```python
from build123d import *

# Parameters (mm, degrees)
SKETCH_W        = 82
SKETCH_H        = 70
PAD_DEPTH       = 2
SKETCH001_W     = 2
SKETCH001_H     = 7
PAD001_DEPTH    = 2
SKETCH011_W     = 8
SKETCH011_H     = 6.8
PAD002_DEPTH    = 4
SKETCH012_W     = 7
SKETCH012_H     = 6
PAD003_DEPTH    = 4
SKETCH010_W     = 8
SKETCH010_H     = 6.8
PAD004_DEPTH    = 4
SKETCH013_R     = 1.15
POCKET_DEPTH    = 80.001
SKETCH016_R     = 1.15
POCKET001_DEPTH = 8.501
SKETCH018_W     = 11.5
SKETCH018_H     = 11.5
POCKET002_DEPTH = 5
POCKET003_DEPTH = 5
POCKET004_DEPTH = 5
SKETCH021_W     = 1
SKETCH021_H     = 7
PAD005_DEPTH    = 1
SKETCH022_W     = 9
SKETCH022_H     = 10
POCKET005_DEPTH = 0.4
FILLET_R        = 2


with BuildPart() as part:
    # Sketch → Pad (new body)
    with BuildSketch(Plane.XY):
        Rectangle(SKETCH_W, SKETCH_H)
    extrude(amount=PAD_DEPTH)

    # Sketch001 (on Face6 of Pad) → Pad001 (join)
    with BuildSketch(Plane.XY.offset(2)):
        with Locations((-38, 0)):
            Rectangle(SKETCH001_W, SKETCH001_H)
        Polygon((-21, 33), (39, 33), (39, -4), (37, -4), (37, 31), (-21, 31), align=None)
    extrude(amount=PAD001_DEPTH)

    # Sketch011 (on Face15 of Pad001) → Pad002 (join)
    with BuildSketch(Plane.YZ.offset(39)):
        with Locations((0, 5.4)):
            Rectangle(SKETCH011_W, SKETCH011_H)
    extrude(amount=-PAD002_DEPTH)

    # Sketch012 (on Face9 of Pad002) → Pad003 (join)
    with BuildSketch(Plane(origin=(-39, 0, 0), x_dir=(0, -1, 0), z_dir=(-1, 0, 0))):
        with Locations((0, 5)):
            Rectangle(SKETCH012_W, SKETCH012_H)
    extrude(amount=-PAD003_DEPTH)

    # Sketch010 (on Face16 of Pad001) → Pad004 (join)
    with BuildSketch(Plane(origin=(0, 33, 0), x_dir=(-1, 0, 0), z_dir=(0, 1, 0))):
        with Locations((-29, 5.4)):
            Rectangle(SKETCH010_W, SKETCH010_H)
        with Locations((14, 5.4)):
            Rectangle(SKETCH010_W, SKETCH010_H)
    extrude(amount=-PAD004_DEPTH)

    # Sketch013 (on Face44 of Pad004) → Pocket (cut, through all)
    with BuildSketch(Plane.YZ.offset(39)):
        with Locations((0, 5)):
            Circle(SKETCH013_R)
    extrude(amount=-POCKET_DEPTH, mode=Mode.SUBTRACT)

    # Sketch016 → Pocket001 (cut, through all)
    with BuildSketch(Plane.XZ.offset(-26.5)):
        with Locations((-14, 5)):
            Circle(SKETCH016_R)
        with Locations((29, 5)):
            Circle(SKETCH016_R)
    extrude(amount=-POCKET001_DEPTH, mode=Mode.SUBTRACT)

    # Sketch018 (on Face5 of Pocket001) → Pocket002 (cut)
    with BuildSketch(Plane.XY.offset(2)):
        with Locations((0, 17.75)):
            Rectangle(SKETCH018_W, SKETCH018_H)
    extrude(amount=-POCKET002_DEPTH, mode=Mode.SUBTRACT)

    # Sketch019 (on Face31 of Pocket002) → Pocket003 (cut)
    with BuildSketch(Plane.XZ.offset(-29)):
        Polygon((29.125944, 9.042901), (33.258869, 4.499726), (33.258869, 9.042901), align=None)
    extrude(amount=-POCKET003_DEPTH, mode=Mode.SUBTRACT)

    # Sketch020 (on Face36 of Pocket003) → Pocket004 (cut)
    with BuildSketch(Plane(origin=(35, 0, 0), x_dir=(0, -1, 0), z_dir=(-1, 0, 0))):
        Polygon((2.77547, 8.938441), (6.386171, 3.079567), (6.386171, 8.938441), align=None)
    extrude(amount=-POCKET004_DEPTH, mode=Mode.SUBTRACT)

    # Sketch021 (on Face40 of Pocket004) → Pad005 (join)
    with BuildSketch(Plane.XY.offset(8)):
        with Locations((-38.5, 0)):
            Rectangle(SKETCH021_W, SKETCH021_H)
    extrude(amount=PAD005_DEPTH)

    # Sketch022 (on Face5 of Pocket003) → Pocket005 (cut)
    with BuildSketch(Plane.XY.offset(2)):
        with Locations((-29.3, 30)):
            Rectangle(SKETCH022_W, SKETCH022_H)
    extrude(amount=-POCKET005_DEPTH, mode=Mode.SUBTRACT)

    # Fillet
    fillet_edges = [part.edges().sort_by_distance(p)[0] for p in [
        (41, 35, 1),
        (-41, 35, 1),
    ]]
    fillet(fillet_edges, radius=FILLET_R)


solid = part.part
```
The model under review builds one solid part; all positions refer to its coordinate system, in mm. A direction names the side the tool comes from. Round coordinates to 2 decimals unless told otherwise and drop trailing zeros. Loops run counter-clockwise (first coordinate to the right, second up) from the corner with the lowest first, then second, coordinate; pieces in that order, holes last.
1) Consider section A-A on x = -14. State the section outline as (y, z) points, then the cut area to 3 significant figures.
Values follow:
outline: (-35, 0) - (35, 0) - (35, 2) - (33, 2) - (33, 3.85) - (29, 3.85) - (29, 2) - (-35, 2) - close; (29, 6.15) - (33, 6.15) - (33, 8.8) - (29, 8.8) - close
area: 158 mm2
2) The part is to be moulded in two halves that separate along Y. For faces 1 (the face through (37, 4, 6)), 2 (the face through (40.4, 34.43, 1.01)), 3 (the face through (8, 32, 4)), say which applies: pulls with the +Y half, pulls with the -Y half, needs draft (parallel to the pull), parting line crosses it, or undercut.
Values follow:
face 1: undercut
face 2: pulls with the +Y half
face 3: needs draft
3) Tool access review of faces 4 (the face through (35, 1, 6)), 5 (the face through (5.75, 18, 1)), 6 (the face through (-19, 32, 4)), 7 (the face through (-29, 30, 1.6)): name each direction out of +Z, -Z, +X, -X, +Y, -Y from which nothing blocks a thin tool from reaching the whole face with its end or side.
Values follow:
face 4: +Z, -Y
face 5: +Z, -Z
face 6: +Z, -X, +Y, -Y
face 7: +Z, +Y
4) Clearance check with flat-ended pins moving along their axes: P1, Ø5, axis at x = -0.5, z = 7.5, coming from the -Y side; P2, Ø1, axis at y = 13.5, z = 3, coming from the -X side; P3, Ø3.5, axis at y = 0, z = 5, coming from the +X side; P4, Ø4.5, axis at x = -16, y = 30.5, coming from the +Z side. State where each tip first meets the part, or that it passes through.
Values follow:
P1: passes through
P2: stops at x = 37
P3: stops at x = 39
P4: stops at z = 8.8
5) Consider section C-C on x = 24. State the section outline as (y, z) points.
Values follow:
outline: (-35, 0) - (35, 0) - (35, 2) - (33, 2) - (33, 4) - (31, 4) - (31, 2) - (-35, 2) - close
6) Wall thickness on line 1 along Z through (x, y) = (-37.75, 0); line 2 along Z through (x, y) = (37.8, 0); line 3 along Y through (x, z) = (-12.5, 4): over which ranges is each line inside the solid? List them lowest first.
Values follow:
line 1: z = 0 to 3.85, 6.15 to 8
line 2: z = 0 to 3.85, 6.15 to 8.8
line 3: y = 29 to 33
7) Consider section B-B on y = 28. State the section outline as (x, z) points, then the cut area to 3 significant figures.
Values follow:
outline: (-41, 0) - (41, 0) - (41, 2) - (39, 2) - (39, 4) - (37, 4) - (37, 2) - (-24.8, 2) - (-24.8, 1.6) - (-33.8, 1.6) - (-33.8, 2) - (-41, 2) - close
area: 164 mm2
8) Consider section D-D on x = -32. State the section outline as (y, z) points.
Values follow:
outline: (-35, 0) - (35, 0) - (35, 1.6) - (25, 1.6) - (25, 2) - (-35, 2) - close
